```python
from build123d import *

# Parameters (mm, degrees)
F1_DEPTH  = 82.55
F2_W      = 9.525
F2_H      = 1.651
F3_DEPTH  = 12.7
F4_W      = 1.651
F4_H      = 9.652
F5_DEPTH  = 3.048
F6_W      = 1.651
F6_H      = 9.652
F7_DEPTH  = 3.048
F9_DEPTH  = 6.35
F11_DEPTH = 6.35
F13_DEPTH = 3.175
F15_DEPTH = 3.175
F16_W     = 6.3165789474
F16_H     = 7.3904166929
F16_W_2   = 2.6257108653
F17_DEPTH = 31.75
F18_W     = 2.54
F18_H     = 50.8
F19_DEPTH = 27.94
F21_DEPTH = 25.4
F23_DEPTH = 25.4


with BuildPart() as f1:
    # F0 (on Top) → F1 (new body)
    with BuildSketch(Plane.XY):
        with BuildLine():
            ThreePointArc((0, 2.54), (0.7439487758, 0.7439487758), (2.54, 0))
            Line((2.54, 0), (48.26, 0))
            ThreePointArc((48.26, 0), (50.0560512242, 0.7439487758), (50.8, 2.54))
            Line((50.8, 2.54), (50.8, 22.86))
            ThreePointArc((50.8, 22.86), (50.0560512242, 24.6560512242), (48.26, 25.4))
            Line((48.26, 25.4), (2.54, 25.4))
            ThreePointArc((2.54, 25.4), (0.7439487758, 24.6560512242), (0, 22.86))
            Line((0, 22.86), (0, 2.54))
        make_face()
        with BuildLine():
            ThreePointArc((1.651, 21.209), (2.3949487758, 23.0050512242), (4.191, 23.749))
            Line((4.191, 23.749), (46.609, 23.749))
            ThreePointArc((46.609, 23.749), (48.4050512242, 23.0050512242), (49.149, 21.209))
            Line((49.149, 21.209), (49.149, 4.191))
            ThreePointArc((49.149, 4.191), (48.4050512242, 2.3949487758), (46.609, 1.651))
            Line((46.609, 1.651), (4.191, 1.651))
            ThreePointArc((4.191, 1.651), (2.3949487758, 2.3949487758), (1.651, 4.191))
            Line((1.651, 4.191), (1.651, 21.209))
        make_face(mode=Mode.SUBTRACT)
    extrude(amount=F1_DEPTH)

    # F2 (on face) → F3 (join)
    with BuildSketch(Plane(origin=(0, 0, 0), x_dir=(1, 0, 0), z_dir=(0, 0, -1))):
        with Locations((30.1625, -0.8255)):
            Rectangle(F2_W, F2_H)
        with Locations((30.1625, -24.5745)):
            Rectangle(F2_W, F2_H)
    extrude(amount=F3_DEPTH)

    # F4 (on face) → F5 (join)
    with BuildSketch(Plane.YZ.offset(34.925)):
        with Locations((0.8255, -7.874)):
            Rectangle(F4_W, F4_H)
    extrude(amount=F5_DEPTH)

    # F6 (on face) → F7 (join)
    with BuildSketch(Plane.YZ.offset(34.925)):
        with Locations((24.5745, -7.874)):
            Rectangle(F6_W, F6_H)
    extrude(amount=F7_DEPTH)

    # F8 (on face) → F9 (cut)
    with BuildSketch(Plane.XZ):
        Polygon((37.973, -12.7), (37.973, -3.048), (25.4, -12.7), align=None)
    extrude(amount=-F9_DEPTH, mode=Mode.SUBTRACT)

    # F10 (on face) → F11 (cut)
    with BuildSketch(Plane(origin=(0, 25.4, 0), x_dir=(-1, 0, 0), z_dir=(0, 1, 0))):
        Polygon((-25.4, -12.7), (-37.973, -3.048), (-37.973, -12.7), align=None)
    extrude(amount=-F11_DEPTH, mode=Mode.SUBTRACT)

    # F12 (on face) → F13 (cut)
    with BuildSketch(Plane(origin=(0, 25.4, 0), x_dir=(-1, 0, 0), z_dir=(0, 1, 0))):
        Polygon((-25.4, -6.096), (-34.0025789474, -6.096), (-25.4, -12.7), align=None)
    extrude(amount=-F13_DEPTH, mode=Mode.SUBTRACT)

    # F14 (on face) → F15 (cut)
    with BuildSketch(Plane.XZ):
        Polygon((25.4, -12.7), (34.6021804274, -5.6356998739), (25.4, -5.6356998739), align=None)
    extrude(amount=-F15_DEPTH, mode=Mode.SUBTRACT)

    # F16 (on face) → F17 (cut)
    with BuildSketch(Plane.XZ):
        with Locations((45.1017105263, 3.6952083465)):
            Rectangle(F16_W, F16_H)
        with Locations((49.5728554326, 3.6952083465)):
            Rectangle(F16_W_2, F16_H)
    extrude(amount=-F17_DEPTH, mode=Mode.SUBTRACT)

    # F18 (on face) → F19 (cut)
    with BuildSketch(Plane.XZ):
        with BuildLine():
            Line((38.1, 25.4), (48.26, 25.4))
            Line((48.26, 25.4), (48.26, 76.2))
            Line((48.26, 76.2), (38.1, 76.2))
            ThreePointArc((38.1, 76.2), (20.1394877579, 68.7605122421), (12.7, 50.8))
            ThreePointArc((12.7, 50.8), (20.1394877579, 32.8394877579), (38.1, 25.4))
        make_face()
        with Locations((49.53, 50.8)):
            Rectangle(F18_W, F18_H)
    extrude(amount=-F19_DEPTH, mode=Mode.SUBTRACT)

    # F20 (on face) → F21 (cut)
    with BuildSketch(Plane(origin=(0, 25.4, 0), x_dir=(-1, 0, 0), z_dir=(0, 1, 0))):
        Polygon((-25.4, -3.048), (-29.7012894737, -6.096), (-25.4, -6.096), align=None)
        Polygon((-41.9434210526, 0), (-38.1, 0), (-41.9434210526, 4.2154166929), align=None)
    extrude(amount=-F21_DEPTH, mode=Mode.SUBTRACT)

    # F22 (on face) → F23 (cut)
    with BuildSketch(Plane(origin=(0, 25.4, 0), x_dir=(-1, 0, 0), z_dir=(0, 1, 0))):
        with BuildLine():
            ThreePointArc((-19.05, 82.55), (-5.5796158184, 76.9703841816), (0, 63.5))
            Line((0, 63.5), (0, 82.55))
            Line((0, 82.55), (-19.05, 82.55))
        make_face()
    extrude(amount=-F23_DEPTH, mode=Mode.SUBTRACT)


solid = f1.part
```
Here's how the part is built. I have some questions about the finished solid (model axes, mm). A direction names the side the tool comes from. Give positions to 0.01 mm unless a question says otherwise; leave off trailing zeros. Order: outer loops, then holes, each group sorted by start corner. A loop starts at its lowest first (then second) coordinate and runs counter-clockwise, first axis right, second up. Notation, with made-up numbers: M -9.5,77 L 10.5,77 A24 cw 10.5,89 Z; hole C -12.5,73 d9. An arc over 180 degrees is marked long. Use a Markdown table: item, result. Add a question column.
1. If we mould it in two halves opening along Y, with no side actions, what happens to faces 6 (the flat face through (36.311, 0.814, -4.324)), 7 (the cylindrical face through (2.41, 2.38, 37.18)), 8 (the cylindrical face through (0.724, 0.764, 35.991))? For each: +Y half, -Y half, draft (parallel to the pull), parting line (faces both ways), or undercut.
2. Suppose I cut it at B-B (x = 11). List the corners of the cut face in (y, z) for me.
3. On a 3-axis mill with a long thin cutter (end or side, diameter ignored), from which of +Z, -Z, +X, -X, +Y, -Y can I reach the whole of each face in a straight line? I mean faces 1 (the flat face through (41.943, 1, 6)), 2 (the flat face through (34.925, 25, -2)), 3 (the flat face through (50.8, 13, 79)), 4 (the flat face through (32, 1, -5.636)), 5 (the flat face through (15.7, 1.651, 37.8)). Say none if no direction works.
4. Suppose I cut it at D-D (x = 32). List the corners of the cut face in (y, z) for me.
5. For pin 1 Ø0.8 at (y, z) = (24.5, 6.5) entering from +X; pin 2 Ø1.3 at (x, y) = (36, 24.5) entering from -Z; pin 3 Ø8.5 at (y, z) = (10, 35.5) entering from +X; pin 4 Ø3 at (x, y) = (24, 5) entering from +Z, each with a flat end and sliding along its axis, tell me the tip position at first contact or that it passes through.
6. Suppose I cut it at C-C (z = 10). List the corners of the cut face in (x, y) for me, and give its area (3 significant figures).
7. Suppose I cut it at A-A (y = 6). List the corners of the cut face in (x, z) for me, and give its area (3 significant figures).
8. I need wall thicknesses on probe 1 along Y at (x, z) = (10.5, 48.5); probe 2 along X at (y, z) = (13, 22); probe 3 along X at (y, z) = (18.25, 47). Which ranges of each line are inside material? Lowest first, please. Write a range as from..to.
Results list:
| question | item | result |
|---|---|---|
| 1 | face 6 | draft |
| 1 | face 7 | undercut |
| 1 | face 8 | -Y half |
| 2 | outline | M 0,0 L 1.65,0 L 1.65,80.77 L 0,80.77 Z; M 23.75,0 L 25.4,0 L 25.4,80.77 L 23.75,80.77 Z |
| 3 | face 1 | -Z, +X, +Y, -Y |
| 3 | face 2 | +X, +Y, -Y |
| 3 | face 3 | +Z, -Z, +X, +Y, -Y |
| 3 | face 4 | -Z, +X, -X, -Y |
| 3 | face 5 | +Z, -Z |
| 4 | outline | M 0,-5.64 L 1.65,-5.64 L 1.65,26.14 L 0,26.14 Z; M 0,75.46 L 1.65,75.46 L 1.65,82.55 L 0,82.55 Z; M 23.75,-6.1 L 25.4,-6.1 L 25.4,26.14 L 23.75,26.14 Z; M 23.75,75.46 L 25.4,75.46 L 25.4,82.55 L 23.75,82.55 Z |
| 5 | pin 1 | stops at x = 41.94 |
| 5 | pin 2 | stops at z = -5.06 |
| 5 | pin 3 | stops at x = 1.65 |
| 5 | pin 4 | passes through |
| 6 | outline | M 0,2.54 A2.54 ccw 2.54,0 L 48.26,0 A2.54 ccw 50.8,2.54 L 50.8,22.86 A2.54 ccw 48.26,25.4 L 2.54,25.4 A2.54 ccw 0,22.86 Z; hole M 1.65,4.19 A2.54 ccw 4.19,1.65 L 46.61,1.65 A2.54 ccw 49.15,4.19 L 49.15,21.21 A2.54 ccw 46.61,23.75 L 4.19,23.75 A2.54 ccw 1.65,21.21 Z |
| 6 | area | 241 mm² |
| 7 | outline | M 0,0 L 1.65,0 L 1.65,71.26 A19.05 ccw 0,63.5 Z; M 49.15,7.39 L 50.8,7.39 L 50.8,25.4 L 49.15,25.4 Z; M 49.15,76.2 L 50.8,76.2 L 50.8,82.55 L 49.15,82.55 Z |
| 7 | area | 154 mm² |
| 8 | probe 1 | y = 0..1.65, 23.75..25.4 |
| 8 | probe 2 | x = 0..1.65, 49.15..50.8 |
| 8 | probe 3 | x = 0..1.65 |
